Design review of the part built by this model. Coordinates are the model's own, in mm. Face numbers are marked on the shaded views. Give positions to 0.01 mm unless a question says otherwise; leave off trailing zeros. Loops run counter-clockwise (first coordinate to the right, second up) from the corner with the lowest first, then second, coordinate; pieces in that order, holes last. Notation, with made-up numbers: M 88,48 L 146,48 A17 ccw 146,53 Z; hole C 20.5,22.5 d6. An arc over 180 degrees is marked long. Answer as CSV lines item,"result".
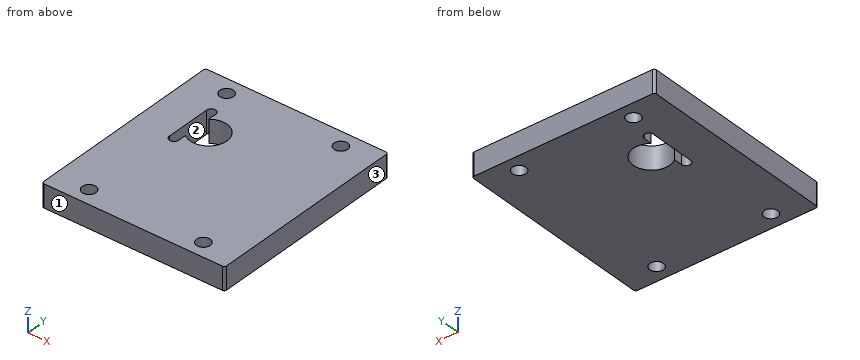
```python
from build123d import *

# Parameters (mm, degrees)
SKETCH_W    = 80
SKETCH_H    = 88
SKETCH_R    = 3
PAD_DEPTH   = 10
FILLET_R    = 1
FILLET001_R = 1


with BuildPart() as part:
    # Sketch → Pad (new body)
    with BuildSketch(Plane.XY):
        with Locations((15, -15)):
            Rectangle(SKETCH_W, SKETCH_H)
        with Locations((-10, -52)):
            Circle(SKETCH_R, mode=Mode.SUBTRACT)
        with Locations((40, -52)):
            Circle(SKETCH_R, mode=Mode.SUBTRACT)
        with Locations((40, 22)):
            Circle(SKETCH_R, mode=Mode.SUBTRACT)
        with Locations((-10, 22)):
            Circle(SKETCH_R, mode=Mode.SUBTRACT)
        with BuildLine():
            ThreePointArc((-5, -6.244998), (8, 0), (-5, 6.244998))
            Line((-5, 6.244998), (-5, 10))
            ThreePointArc((-5, 10), (-7, 12), (-9, 10))
            Line((-9, 10), (-9, -10))
            ThreePointArc((-9, -10), (-7, -12), (-5, -10))
            Line((-5, -6.244998), (-5, -10))
        make_face(mode=Mode.SUBTRACT)
    extrude(amount=PAD_DEPTH)

    # Fillet
    fillet_edges = [part.edges().sort_by_distance(p)[0] for p in [
        (-25, -59, 5),
        (-25, 29, 5),
    ]]
    fillet(fillet_edges, radius=FILLET_R)

    # Fillet001
    fillet001_edges = [part.edges().sort_by_distance(p)[0] for p in [
        (55, -59, 5),
        (55, 29, 5),
    ]]
    fillet(fillet001_edges, radius=FILLET001_R)


solid = part.part
```
1. We need section D-D, the plane x = 1. Write out the cut boundary in (y, z), plus the area to 3 significant figures.
Answer block:
outline,"M -59,0 L -7.94,0 L -7.94,10 L -59,10 Z; M 7.94,0 L 29,0 L 29,10 L 7.94,10 Z"
area,"721 mm²"
2. We need section B-B, the plane z = 1.75. Write out the cut boundary in (x, y) (3 decimals), plus the area to 3 significant figures.
Answer block:
outline,"M -25,-58 A1 ccw -24,-59 L 54,-59 A1 ccw 55,-58 L 55,28 A1 ccw 54,29 L -24,29 A1 ccw -25,28 Z; hole C -10,-52 d6; hole C -10,22 d6; hole M -9,-10 A2 ccw -5,-10 L -5,-6.245 A8 ccw long -5,6.245 L -5,10 A2 ccw -9,10 Z; hole C 40,-52 d6; hole C 40,22 d6"
area,"6,660 mm²"
3. To check wall thickness, follow L1, parallel to Y at x = -10, z = 7.25; L2, parallel to X at y = 0, z = 4; L3, parallel to Y at x = -11, z = 9.5. State the ranges of each line that lie inside material, in increasing order. Write a range as [from, to].
Answer block:
L1,"[-59, -55], [-49, 19], [25, 29]"
L2,"[-25, -9], [8, 55]"
L3,"[-59, -54.83], [-49.17, 19.17], [24.83, 29]"
4. We need section A-A, the plane y = -4. Write out the cut boundary in (x, z), plus the area to 3 significant figures.
Answer block:
outline,"M -25,0 L -9,0 L -9,10 L -25,10 Z; M 6.93,0 L 55,0 L 55,10 L 6.93,10 Z"
area,"641 mm²"
5. The part is to be moulded in two halves that separate along Y. For the marked faces 1, 2 and 3, say which applies: pulls with the +Y half, pulls with the -Y half, needs draft (parallel to the pull), parting line crosses it, or undercut.
Answer block:
face 1,"pulls with the -Y half"
face 2,"undercut"
face 3,"needs draft"
6. We need section C-C, the plane y = 22. Write out the cut boundary in (x, z), plus the area to 3 significant figures.
Answer block:
outline,"M -25,0 L -13,0 L -13,10 L -25,10 Z; M -7,0 L 37,0 L 37,10 L -7,10 Z; M 43,0 L 55,0 L 55,10 L 43,10 Z"
area,"680 mm²"
